The model under review builds one solid part; all positions refer to its coordinate system, in mm. Face numbers are marked on the shaded views. Round coordinates to 2 decimals unless told otherwise and drop trailing zeros. Write each loop counter-clockwise with the first axis right and the second up, starting at its lowest first coordinate (ties: lowest second). Pieces come first, ordered by that corner, then holes. Notation, with made-up numbers: (11, 44) -> (21, 44) arc R27 ccw to (21, 69) -> close; hole circle Ø5 at (82, -12.5). An arc over 180 degrees is marked (long way). Return JSON: item names as keys, results as strings. Group by question number.
1. For line 1 along X through (y, z) = (-1.25, 5.75); line 2 along Y through (x, z) = (-0.75, 6.65); line 3 along Y through (x, z) = (0.25, 5.95), list the stretches that pass through material, from the lowest coordinate up. Write a range as from..to.
2. Mouldability with a two-part tool opening along X and no side actions: class the marked faces 1, 2, 3 and 4 as pulls with the +X half, pulls with the -X half, needs draft (parallel to the pull), parting line crosses it, or undercut.
3. Take a section at A-A, the plane z = 6.7. Write out the cut boundary in (x, y), then the cut area to 3 significant figures.
from build123d import *

# Parameters (mm, degrees)
SKETCH013_R     = 8.20375
POCKET004_DEPTH = 5
CHAMFER001_SIZE = 0.25


with BuildPart() as part:
    # Sketch012 → Revolution001 (revolve)
    with BuildSketch(Plane.XZ):
        Polygon((2.9, 0.875), (2.9, -0.875), (3.9, -0.875), (7.165544, 0), (3.9, 0.875), align=None)
    revolve(axis=Axis((0, 0, 0), (0, 0, 1)))

    # Sketch013 (on Face5 of Revolution001) → Pocket004 (cut)
    with BuildSketch(Plane(origin=(0, 0, 0.875), x_dir=(-1, 0, 0), z_dir=(0, 0, 1))):
        Circle(SKETCH013_R)
        Polygon((0, 4.503332), (-3.9, 2.251666), (-3.9, -2.251666), (0, -4.503332), (3.9, -2.251666), (3.9, 2.251666), align=None, mode=Mode.SUBTRACT)
    extrude(amount=-POCKET004_DEPTH, mode=Mode.SUBTRACT)

    # Chamfer001
    chamfer001_edges = [part.edges().sort_by_distance(p)[0] for p in [
        (-2.9, 0, -0.875),
        (-2.9, 0, 0.875),
    ]]
    chamfer(chamfer001_edges, length=CHAMFER001_SIZE)


with BuildPart() as part_1:
    # Body003 placement: moved
    add(part.part.moved(Location((0, 0, 0.875))))


with BuildPart() as part_2:
    # Body004 placement: moved
    add(part_1.part.moved(Location((0, 0, 5.35))))


solid = part_2.part
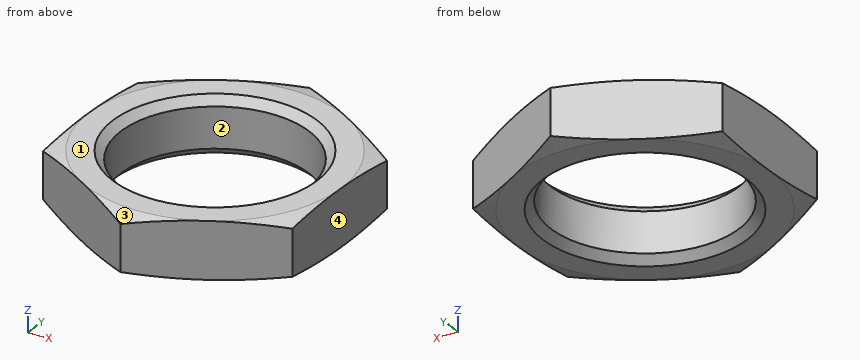
Output:
{
 "1": {"line 1": "x = -3.9..-2.62, 2.62..3.9", "line 2": "y = -4.07..-2.8, 2.8..4.07", "line 3": "y = -4.36..-2.89, 2.89..4.36"},
 "2": {"face 1": "needs draft", "face 2": "undercut", "face 3": "parting line crosses it", "face 4": "pulls with the +X half"},
 "3": {"outline": "(-3.9, -2.25) -> (0, -4.5) -> (3.9, -2.25) -> (3.9, 2.25) -> (0, 4.5) -> (-3.9, 2.25) -> close; hole circle Ø5.8 at (0, 0)", "area": "26.3 mm^2"}
}
